```python
from build123d import *

# Parameters (mm, degrees)
F0_R     = 50
F1_DEPTH = 60
F3_DEPTH = 80
F4_W     = 50
F4_H     = 50
F5_DEPTH = 140


with BuildPart() as f1:
    # F0 (on Top) → F1 (new body)
    with BuildSketch(Plane.XY):
        Circle(F0_R)
    extrude(amount=F1_DEPTH)

    # F2 (on face) → F3 (cut)
    with BuildSketch(Plane.XY.offset(60)):
        with BuildLine():
            Line((0, -50), (0, 0))
            Line((0, 0), (-50, 0))
            ThreePointArc((-50, 0), (-35.355339, -35.355339), (0, -50))
        make_face()
    extrude(amount=-F3_DEPTH, mode=Mode.SUBTRACT)

    # F4 (on Top) → F5 (join)
    with BuildSketch(Plane.XY):
        with Locations((-25, -25)):
            Rectangle(F4_W, F4_H)
    extrude(amount=F5_DEPTH)


solid = f1.part
```
Input: part model. Units: mm. Frame: model coordinates. A direction names the side the tool comes from. Round coordinates to 2 decimals unless told otherwise and drop trailing zeros. Loops run counter-clockwise (first coordinate to the right, second up) from the corner with the lowest first, then second, coordinate; pieces in that order, holes last. Notation, with made-up numbers: (51, -27) - (89, -27) arc R38 cw to (89, 12) - close; hole circle Ø4 at (-18, 7.25). An arc over 180 degrees is marked (long way). One line per item, written item: value. Start each with the question number.
(1) Section C-C, the plane y = 9. Return loops of the section in (x, z), plus the area to 3 significant figures.
(2) Section B-B, the plane z = 46.5. Return loops of the section in (x, y), plus the area to 3 significant figures.
(3) Contact query for flat-ended pins moving along their axis: P1, Ø10, axis at x = 0.5, z = 37.5, coming from the +Y side; P2, Ø8, axis at y = 21, z = 52, coming from the +X side; P3, Ø10, axis at x = 17, y = 27, coming from the +Z side. Output: stop coordinate, or through.
(4) Ray query, line 1 (X direction, y = -10.5, z = 88.5); line 2 (Z direction, x = -18, y = 2.5). Return the intervals inside material, ascending. Write a range as [from, to].
(5) Section D-D, the plane z = 130. Return loops of the section in (x, y), plus the area to 3 significant figures.
(6) Section A-A, the plane x = -30. Return loops of the section in (y, z).
(7) Access query for faces 1 (the cylindrical face through (36.5, 34.17, 29.58)), 2 (the flat face through (-25, 0, 99)), 3 (the flat face through (0, -25, 99)). Directions: +Z, -Z, +X, -X, +Y, -Y. A direction counts if a zero-diameter tool reaches every point of the face in a straight line with its end or side. Return the directions, or none.
Results below:
1. outline: (-49.18, 0) - (49.18, 0) - (49.18, 60) - (-49.18, 60) - close
1. area: 5,900 mm^2
2. outline: (-50, -50) - (0, -50) arc R50 ccw (long way) to (-50, 0) - close
2. area: 8,390 mm^2
3. P1: y = 50
3. P2: x = 47.02
3. P3: z = 60
4. line 1: [-50, 0]
4. line 2: [0, 60]
5. outline: (-50, -50) - (0, -50) - (0, 0) - (-50, 0) - close
5. area: 2,500 mm^2
6. outline: (-50, 0) - (40, 0) - (40, 60) - (0, 60) - (0, 140) - (-50, 140) - close
7. face 1: +Z, -Z
7. face 2: +Z, +X, -X, +Y
7. face 3: +Z, +X, +Y, -Y
